from build123d import *

# Parameters (mm, degrees)
F0_R     = 5.3975
F1_DEPTH = 6.35
F2_R     = 4.0005
F3_DEPTH = 3.429
F4_R     = 4.0005
F5_DEPTH = 3.429


with BuildPart() as f1:
    # F0 (on Top) → F1 (new body, symmetric)
    with BuildSketch(Plane.XY):
        Circle(F0_R)
    extrude(amount=F1_DEPTH, both=True)

    # F2 (on face) → F3 (join)
    with BuildSketch(Plane(origin=(0, 0, -6.35), x_dir=(1, 0, 0), z_dir=(0, 0, -1))):
        Circle(F2_R)
    extrude(amount=F3_DEPTH)

    # F4 (on face) → F5 (join)
    with BuildSketch(Plane.XY.offset(6.35)):
        Circle(F4_R)
    extrude(amount=F5_DEPTH)


solid = f1.part
Can you work these out from the model? Positions are in its coordinate system, mm. A direction names the side the tool comes from. Give positions to 0.01 mm unless a question says otherwise; leave off trailing zeros. Loops run counter-clockwise (first coordinate to the right, second up) from the corner with the lowest first, then second, coordinate; pieces in that order, holes last. Notation, with made-up numbers: (64, -6) - (108, -6) arc R4 cw to (108, 0) - close; hole circle Ø5 at (78, -22). An arc over 180 degrees is marked (long way). Answer as a JSON object with one key per item and string values.
Q1. Will these pins go through, and if not, where does the flat tip stop? P1, Ø1.5, axis at y = -1, z = 3, coming from the -X side; P2, Ø5, axis at y = -3, z = 4.5, coming from the +X side; P3, Ø5, axis at x = 0.5, z = -2.5, coming from the +Y side; P4, Ø5, axis at y = 3.5, z = -2, coming from the +X side.
Geometry says:
{"P1": "x = -5.39", "P2": "x = 5.37", "P3": "y = 5.4", "P4": "x = 5.3"}
Q2. If I drill on L1, parallel to Z at x = 3.75, y = -3.75; L2, parallel to Y at x = 0, z = -9; L3, parallel to X at y = -4, z = -1, over which ranges is the centre line in solid material (lowest first)?
Geometry says:
{"L1": "-6.35 to 6.35", "L2": "-4 to 4", "L3": "-3.62 to 3.62"}
Q3. Imagine slicing it at D-D on z = 5.25. Write out the boundary of the cut face in (x, y) (1 decimal), plus the area to 3 significant figures.
Geometry says:
{"outline": "circle Ø10.8 at (0, 0)", "area": "91.5 mm²"}
Q4. Imagine slicing it at A-A on y = 0. Write out the boundary of the cut face in (x, z), plus the area to 3 significant figures.
Geometry says:
{"outline": "(-5.4, -6.35) - (-4, -6.35) - (-4, -9.78) - (4, -9.78) - (4, -6.35) - (5.4, -6.35) - (5.4, 6.35) - (4, 6.35) - (4, 9.78) - (-4, 9.78) - (-4, 6.35) - (-5.4, 6.35) - close", "area": "192 mm²"}
Q5. Imagine slicing it at C-C on z = 8.5. Write out the boundary of the cut face in (x, y), plus the area to 3 significant figures.
Geometry says:
{"outline": "circle Ø8 at (0, 0)", "area": "50.3 mm²"}
Q6. Which directions (+Z, -Z, +X, -X, +Y, -Y) give clear straight access to the entire face, cutting with the end or side of a thin tool? Please do faces 1 (the flat face through (-4, -2, 6.35)), 2 (the flat face through (-4, -2, -6.35)), 3 (the flat face through (0, 0, -9.779)).
Geometry says:
{"face 1": "+Z", "face 2": "-Z", "face 3": "-Z, +X, -X, +Y, -Y"}
